```python
from build123d import *

# Parameters (mm, degrees)
DODANIE_WYCI_GNI_CIE1_DEPTH = 10
SKALA1_SCALE                = 0.9


with BuildPart() as part:
    # Szkic1 → Dodanie-wyciągnięcie1 (new body)
    with BuildSketch(Plane.XY):
        with BuildLine():
            ThreePointArc((-4.61531313, 22.743178996), (-18.644238864, 25.090860352), (-26.425868288, 13.184197993))
            ThreePointArc((-26.425868288, 13.184197993), (-19.794080105, -8.974802604), (-1.896314698, -23.62648904))
            ThreePointArc((-1.896314698, -23.62648904), (0, -24.000044339), (1.896314698, -23.62648904))
            ThreePointArc((1.896314698, -23.62648904), (19.794080105, -8.974802604), (26.425868288, 13.184197993))
            ThreePointArc((26.425868288, 13.184197993), (18.644238864, 25.090860352), (4.61531313, 22.743178996))
            ThreePointArc((4.61531313, 22.743178996), (3.856622065, 22.481767555), (3.150062494, 22.862190539))
            ThreePointArc((3.150062494, 22.862190539), (0, 24.397011786), (-3.150062494, 22.862190539))
            ThreePointArc((-3.150062494, 22.862190539), (-3.856622065, 22.481767555), (-4.61531313, 22.743178996))
        make_face()
    extrude(amount=DODANIE_WYCI_GNI_CIE1_DEPTH)


with BuildPart() as part_1:
    # Skala1: scaled about (0, 3.998335482, 5)
    add(part.part.scale(SKALA1_SCALE).moved(Location((0, 0.399833548, 0.5))))


solid = part_1.part
```
For this review, take the finished solid that the model builds, in its own axes (mm). Coordinates: 2 decimals unless noted, no trailing zeros. Order: outer loops, then holes, each group sorted by start corner. A loop starts at its lowest first (then second) coordinate and runs counter-clockwise, first axis right, second up. Notation, with made-up numbers: (10, 36.25) -> (53, 36.25) arc R31 ccw to (53, 60.25) -> close; hole circle Ø11 at (81.25, 26). An arc over 180 degrees is marked (long way). Answer as CSV lines item,"result".
Q1. Wall thickness on line 1 along X through (y, z) = (21, 2.5); line 2 along Y through (x, z) = (-18, 2); line 3 along Y through (x, z) = (-18.5, 6.75): over which ranges is each line inside the solid? List them lowest first. Write a range as [from, to].
Model answer:
line 1,"x = [-19.87, -4.3], [-2.82, 2.82], [4.3, 19.87]"
line 2,"y = [-7.4, 22.36]"
line 3,"y = [-6.61, 22.05]"
Q2. Clearance check with flat-ended pins moving along their axes: pin 1 Ø2 at (y, z) = (-3, 6) entering from -X; pin 2 Ø3 at (y, z) = (-12, 2) entering from -X; pin 3 Ø4 at (x, z) = (-12, 6) entering from -Y. State where each tip first meets the part, or that it passes through.
Model answer:
pin 1,"stops at x = -20.89"
pin 2,"stops at x = -15.73"
pin 3,"stops at y = -16.07"
Q3. We need section C-C (x = -15.5). State the section outline as (y, z) points.
Model answer:
outline,"(-10.77, 0.5) -> (23.46, 0.5) -> (23.46, 9.5) -> (-10.77, 9.5) -> close"
Q4. We need section A-A (z = 7.25). State the section outline as (x, y) points.
Model answer:
outline,"(-23.78, 12.27) arc R35.57 ccw to (-1.71, -20.86) arc R4.5 ccw to (1.71, -20.86) arc R35.57 ccw to (23.78, 12.27) arc R11.7 ccw to (4.15, 20.87) arc R0.9 cw to (2.84, 20.98) arc R3.6 ccw to (-2.84, 20.98) arc R0.9 cw to (-4.15, 20.87) arc R11.7 ccw to start"
Q5. We need section B-B (y = -5). State the section outline as (x, z) points.
Model answer:
outline,"(-19.43, 0.5) -> (19.43, 0.5) -> (19.43, 9.5) -> (-19.43, 9.5) -> close"
